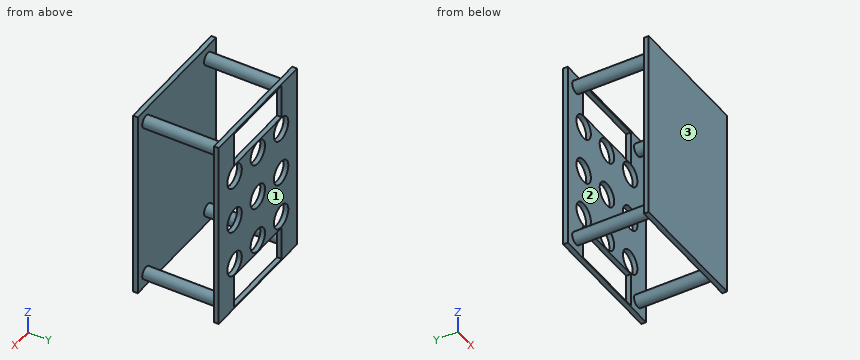
Autodesk Inventor part; units mm, degrees
ref_plane "YZ Plane" through (0, 0, 0) normal (1, 0, 0) x (0, 1, 0)
ref_plane "XZ Plane" through (0, 0, 0) normal (0, 1, 0) x (-1, 0, 0)
ref_plane "XY Plane" through (0, 0, 0) normal (0, 0, 1) x (1, 0, 0)
sketch "Sketch1" plane through (0, 0, 0) normal (0, 1, 0) x (-1, 0, 0)
  line L0 (0, 0) -> (85.48, 0)
  line L1 (85.48, 0) -> (85.48, -127.76)
  line L2 (85.48, -127.76) -> (0, -127.76)
  line L3 (0, -127.76) -> (0, 0)
  dimension "d0" = 85.48
  dimension "d1" = 127.76
extrude "Extrusion1" add sketch "Sketch1" along normal blind 3.175
sketch "Sketch2" plane through (0, 3.175, 0) normal (0, 1, 0) x (1, 0, 0)
  line L0 (0, 0) -> (-8.9803, 8.9803)
  line L1 (-85.48, 127.76) -> (-85.48, 0)
  line L2 (-85.48, 0) -> (-76.4997, 8.9803)
  line L3 (-85.48, 0) -> (-72.78, 0) construction
  line L4 (0, 127.76) -> (-85.48, 127.76)
  line L5 (-85.48, 127.76) -> (-76.4997, 118.7797)
  line L6 (-85.48, 127.76) -> (-72.78, 127.76) construction
  line L7 (0, 127.76) -> (-8.9803, 118.7797)
  circle A0 centre (-76.4997, 118.7797) radius 4.1275
  circle A1 centre (-8.9803, 118.7797) radius 4.1275
  circle A2 centre (-76.4997, 8.9803) radius 4.1275
  circle A3 centre (-8.9803, 8.9803) radius 4.1275
  dimension "d4" = 12.7
  dimension "d5" = 12.7
  dimension "d6" = 45
  dimension "d7" = 12.7
  dimension "d8" = 45
  dimension "d9" = 12.7
  dimension "d10" = 8.255
  dimension "d11" = 8.255
  dimension "d12" = 8.255
  dimension "d13" = 8.255
extrude "Extrusion2" add sketch "Sketch2" along normal blind 50.8
sketch "Sketch3" plane through (-76.4997, 53.975, -8.9803) normal (0, 1, 0) x (1, 0, 0)
  line L0 (-8.9803, -8.9803) -> (76.4997, -8.9803)
  line L1 (-8.9803, 118.7797) -> (-8.9803, -8.9803)
  line L2 (76.4997, 118.7797) -> (-8.9803, 118.7797)
  line L3 (76.4997, -8.9803) -> (76.4997, 118.7797)
extrude "Extrusion3" add sketch "Sketch3" along normal blind 3.175
sketch "Sketch4" plane through (-76.4997, 57.15, -8.9803) normal (0, 1, 0) x (1, 0, 0)
  line L0 (-8.9803, -8.9803) -> (76.4997, -8.9803)
  line L1 (33.7597, -8.9803) -> (33.7597, 118.7797)
  line L2 (76.4997, 118.7797) -> (-8.9803, 118.7797)
  line L3 (33.7597, 54.8997) -> (33.7597, 86.6497)
  line L4 (33.7597, 54.8997) -> (65.5097, 54.8997) construction
  line L5 (33.7597, 54.8997) -> (33.7597, 23.1497)
  circle A0 centre (33.7597, 86.6497) radius 7.874
  circle A1 centre (33.7597, 23.1497) radius 7.874
  circle A2 centre (33.7597, 54.8997) radius 7.874
  line L6 (33.7597, 86.6497) -> (59.1597, 86.6497)
  circle A3 centre (59.1597, 86.6497) radius 7.874
  line L7 (33.7597, 86.6497) -> (8.3597, 86.6497)
  line L8 (33.7597, 54.8997) -> (59.1597, 54.8997)
  line L9 (33.7597, 54.8997) -> (8.3597, 54.8997)
  line L10 (33.7597, 23.1497) -> (59.1597, 23.1497)
  line L11 (33.7597, 23.1497) -> (8.3597, 23.1497)
  line L12 (33.7597, 23.1497) -> (59.1597, 23.1497) construction
  circle A4 centre (8.3597, 86.6497) radius 7.874
  circle A5 centre (8.3597, 54.8997) radius 7.874
  circle A6 centre (59.1597, 54.8997) radius 7.874
  circle A7 centre (59.1597, 23.1497) radius 7.874
  circle A8 centre (8.3597, 23.1497) radius 7.874
  line L13 (7.7247, 95.1761) -> (59.7947, 95.1761)
  line L14 (59.7947, 95.1761) -> (59.7947, 118.0361)
  line L15 (59.7947, 118.0361) -> (7.7247, 118.0361)
  line L16 (7.7247, 118.0361) -> (7.7247, 95.1761)
  line L17 (7.7247, 95.1761) -> (59.7947, 118.0361) construction
  line L18 (59.7947, 95.1761) -> (7.7247, 118.0361) construction
  line L19 (7.7247, 15.1012) -> (59.7947, 15.1012)
  line L20 (59.7947, 15.1012) -> (59.7947, -7.7588)
  line L21 (59.7947, -7.7588) -> (7.7247, -7.7588)
  line L22 (7.7247, -7.7588) -> (7.7247, 15.1012)
  line L23 (7.7247, 15.1012) -> (59.7947, -7.7588) construction
  line L24 (59.7947, 15.1012) -> (7.7247, -7.7588) construction
  point P0 (33.7597, 106.6061)
  point P1 (33.7597, 3.6712)
  dimension "d18" = 31.75
  dimension "d19" = 90
  dimension "d20" = 31.75
  dimension "d21" = 15.748
  dimension "d22" = 15.748
  dimension "d25" = 15.748
  dimension "d26" = 25.4
  dimension "d27" = 15.748
  dimension "d28" = 25.4
  dimension "d29" = 25.4
  dimension "d30" = 25.4
  dimension "d31" = 25.4
  dimension "d32" = 25.4
  dimension "d33" = 180
  dimension "d34" = 15.748
  dimension "d35" = 15.748
  dimension "d36" = 15.748
  dimension "d37" = 15.748
  dimension "d38" = 15.748
  dimension "d39" = 52.07
  dimension "d40" = 22.86
  dimension "d41" = 52.07
  dimension "d42" = 22.86
extrude "Extrusion4" cut sketch "Sketch4" against normal blind 3.175
properties part number "Elve tube holder"
Geometry: final body of the model. Coordinates: model frame, mm. Face numbers are marked on the shaded views. Round coordinates to 2 decimals unless told otherwise and drop trailing zeros. Loops run counter-clockwise (first coordinate to the right, second up) from the corner with the lowest first, then second, coordinate; pieces in that order, holes last.
Q1. Section B-B on z = -74. Return loops of the section in (x, y) (3 decimals).
Q2. Pull-direction query (Y, two-part tool) for the marked faces 1, 2 and 3; classes: released by +Y, released by -Y, zero draft, split by the parting line, or undercut.
Q3. Material intervals for L1, parallel to Z at x = -68.14, y = 56.4; L2, parallel to X at y = 55.5, z = -63.88; L3, parallel to Y at x = -76.5, z = -40 (3 decimals), sorted ascending.
Q4. Section D-D on z = -95.63. Return loops of the section in (x, y) (3 decimals).
Q5. Section A-A on x = -42.74. State how many separate pieces and enclosed holes the cut face has, plus the area to 3 significant figures.
Q6. Pin query (flat end, axial travel): P1, Ø5, axis at x = -23, y = 50.5, coming from the -Z side; P2, Ø14, axis at x = -68.14, z = -95.63, coming from the +Y side (3 decimals); P3, Ø3, axis at x = -74, y = 19.5, coming from the +Z side. Return the tip coordinate at first contact, or that it passes through.
Evaluation:
1. outline: (-85.48, 0) - (0, 0) - (0, 3.175) - (-85.48, 3.175) - close; (-85.48, 53.975) - (0, 53.975) - (0, 57.15) - (-85.48, 57.15) - close
2. face 1: released by +Y
2. face 2: undercut
2. face 3: released by -Y
3. L1: z = -127.76 to -127.02, -104.16 to -103.5, -87.76 to -71.75, -56.01 to -40, -24.26 to -24.08, -1.22 to 0
3. L2: x = -85.48 to -76.01, -60.27 to -50.61, -34.87 to -25.21, -9.47 to 0
3. L3: y = 0 to 3.175, 53.975 to 57.15
4. outline: (-85.48, 0) - (0, 0) - (0, 3.175) - (-85.48, 3.175) - close; (-85.48, 53.975) - (-76.014, 53.975) - (-76.014, 57.15) - (-85.48, 57.15) - close; (-60.266, 53.975) - (-50.614, 53.975) - (-50.614, 57.15) - (-60.266, 57.15) - close; (-34.866, 53.975) - (-25.214, 53.975) - (-25.214, 57.15) - (-34.866, 57.15) - close; (-9.466, 53.975) - (0, 53.975) - (0, 57.15) - (-9.466, 57.15) - close
5. separate pieces: 7
5. enclosed holes: 0
5. area: 516 mm2
6. P1: passes through
6. P2: stops at y = 3.175
6. P3: stops at z = -4.98
